Source: CAD feature listing. Evaluate the final solid. Frame: model axes, mm. A direction names the side the tool comes from. Round coordinates to 2 decimals unless told otherwise and drop trailing zeros. Loops run counter-clockwise (first coordinate to the right, second up) from the corner with the lowest first, then second, coordinate; pieces in that order, holes last. Notation, with made-up numbers: (77.25, -19.75) -> (135.25, -19.75) arc R29 ccw to (135.25, 19.25) -> close; hole circle Ø1 at (67, -36). An arc over 180 degrees is marked (long way). Put each result on its own line as item: value. Start each with the question number.
1. Set-up query: faces 4 (the flat face through (-95, -25, 187)), 5 (the flat face through (155, -25, -188)), 6 (the flat face through (-3, 141, -187.5)), 7 (the flat face through (219, 149, -100)), 8 (the flat face through (-125, -41, 175)). Return all of +Z, -Z, +X, -X, +Y, -Y with unobstructed straight access to the full face (end or side cutting, diameter ignored); none if empty.
2. Cut plane B-B (x = 125). Return the cut outline in (y, z), then the cut area to 3 significant figures.
3. Cut plane A-A (y = 305). Return the cut outline in (x, z).
4. Material intervals for L1, parallel to Z at x = 35.5, y = 98.5; L2, parallel to X at y = 119, z = 139; L3, parallel to Y at x = -0.5, z = 0, sorted ascending.
5. Cut plane D-D (z = 0). Return the cut outline in (x, y).
6. Draft query along Z for faces 1 (the flat face through (125, -50, 188)), 2 (the flat face through (0, 188, 15)), 3 (the flat face through (-3, 83, 200)). Return one class per face: pulls with the +Z half, pulls with the -Z half, needs draft (parallel to the pull), parting line crosses it, or undercut.
7. Cut plane C-C (y = -25). State how many separate pieces and enclosed holes the cut face has, then the cut area to 3 significant figures.
8. Contact query for flat-ended pins moving along their axis: pin 1 (23 mm diameter, centred on y = 305, z = 0, fed in from +X); pin 2 (1.5 mm diameter, centred on x = -73.5, z = 112.5, fed in from -Y); pin 3 (7.5 mm diameter, centred on y = -34, z = -188, fed in from +X); pin 4 (25 mm diameter, centred on x = 128.5, y = -19.5, fed in from +Z). Output: stop coordinate, or through.
```python
from build123d import *

# Parameters (mm, degrees)
SKETCH1_W           = 450
SKETCH1_H           = 400
BOSS_EXTRUDE1_DEPTH = 220
SKETCH2_W           = 425
SKETCH2_H           = 375
CUT_EXTRUDE1_DEPTH  = 160
SKETCH3_W           = 200
SKETCH3_H           = 140
CUT_EXTRUDE2_DEPTH  = 12.5
SKETCH4_W           = 30
SKETCH4_H           = 30
BOSS_EXTRUDE2_DEPTH = 260
SKETCH5_R           = 10
CUT_EXTRUDE3_DEPTH  = 30
SKETCH6_W           = 60
SKETCH6_H           = 25
BOSS_EXTRUDE3_DEPTH = 50
SKETCH7_R           = 15
CUT_EXTRUDE4_DEPTH  = 25
SKETCH8_R           = 15
CUT_EXTRUDE5_DEPTH  = 25


with BuildPart() as part:
    # Sketch1 → Boss-Extrude1 (new body)
    with BuildSketch(Plane(origin=(0, 0, 0), x_dir=(1, 0, 0), z_dir=(0, 1, 0))):
        Rectangle(SKETCH1_W, SKETCH1_H)
    extrude(amount=BOSS_EXTRUDE1_DEPTH)

    # Sketch2 → Cut-Extrude1 (cut)
    with BuildSketch(Plane(origin=(0, 220, 0), x_dir=(1, 0, 0), z_dir=(0, 1, 0))):
        Rectangle(SKETCH2_W, SKETCH2_H)
    extrude(amount=-CUT_EXTRUDE1_DEPTH, mode=Mode.SUBTRACT)

    # Sketch3 → Cut-Extrude2 (cut)
    with BuildSketch(Plane(origin=(225, 0, 0), x_dir=(0, 0, -1), z_dir=(1, 0, 0))):
        with Locations((0, 150)):
            Rectangle(SKETCH3_W, SKETCH3_H)
    extrude(amount=-CUT_EXTRUDE2_DEPTH, mode=Mode.SUBTRACT)

    # Sketch4 → Boss-Extrude2 (add)
    with BuildSketch(Plane(origin=(0, 60, 0), x_dir=(1, 0, 0), z_dir=(0, 1, 0))):
        Rectangle(SKETCH4_W, SKETCH4_H)
    extrude(amount=BOSS_EXTRUDE2_DEPTH)

    # Sketch5 → Cut-Extrude3 (cut)
    with BuildSketch(Plane(origin=(15, 0, 0), x_dir=(0, 0, -1), z_dir=(1, 0, 0))):
        with Locations((0, 305)):
            Circle(SKETCH5_R)
    extrude(amount=-CUT_EXTRUDE3_DEPTH, mode=Mode.SUBTRACT)

    # Sketch6 → Boss-Extrude3 (add)
    with BuildSketch(Plane.XZ):
        with Locations((125, 187.5)):
            Rectangle(SKETCH6_W, SKETCH6_H)
        with Locations((-125, 187.5)):
            Rectangle(SKETCH6_W, SKETCH6_H)
        with Locations((-125, -187.5)):
            Rectangle(SKETCH6_W, SKETCH6_H)
        with Locations((125, -187.5)):
            Rectangle(SKETCH6_W, SKETCH6_H)
    extrude(amount=BOSS_EXTRUDE3_DEPTH)

    # Sketch7 → Cut-Extrude4 (cut)
    with BuildSketch(Plane(origin=(0, 0, -200), x_dir=(-1, 0, 0), z_dir=(0, 0, -1))):
        with Locations((125, -25)):
            Circle(SKETCH7_R)
        with Locations((-125, -25)):
            Circle(SKETCH7_R)
    extrude(amount=-CUT_EXTRUDE4_DEPTH, mode=Mode.SUBTRACT)

    # Sketch8 → Cut-Extrude5 (cut)
    with BuildSketch(Plane.XY.offset(200)):
        with Locations((-125, -25)):
            Circle(SKETCH8_R)
        with Locations((125, -25)):
            Circle(SKETCH8_R)
    extrude(amount=-CUT_EXTRUDE5_DEPTH, mode=Mode.SUBTRACT)


solid = part.part
```
Solution:
1. face 4: +Z, -Z, -Y
1. face 5: +Z, -Z, +X, -Y
1. face 6: +Y
1. face 7: +X, +Y
1. face 8: +X, -X, -Y
2. outline: (-50, -200) -> (-40, -200) -> (-40, -175) -> (-50, -175) -> close; (-50, 175) -> (-40, 175) -> (-40, 200) -> (-50, 200) -> close; (-10, -200) -> (220, -200) -> (220, -187.5) -> (60, -187.5) -> (60, 187.5) -> (220, 187.5) -> (220, 200) -> (-10, 200) -> (-10, 175) -> (0, 175) -> (0, -175) -> (-10, -175) -> close
2. area: 29,000 mm^2
3. outline: (-15, -15) -> (15, -15) -> (15, -10) -> (-15, -10) -> close; (-15, 10) -> (15, 10) -> (15, 15) -> (-15, 15) -> close
4. L1: z = -200 to -187.5, 187.5 to 200
4. L2: x = -225 to -212.5, 212.5 to 225
4. L3: y = 0 to 295, 315 to 320
5. outline: (-225, 0) -> (225, 0) -> (225, 80) -> (212.5, 80) -> (212.5, 60) -> (15, 60) -> (15, 295) -> (-15, 295) -> (-15, 60) -> (-212.5, 60) -> (-212.5, 220) -> (-225, 220) -> close; (-15, 315) -> (15, 315) -> (15, 320) -> (-15, 320) -> close
6. face 1: needs draft
6. face 2: undercut
6. face 3: pulls with the +Z half
7. separate pieces: 8
7. enclosed holes: 0
7. area: 3,000 mm^2
8. pin 1: stops at x = 15
8. pin 2: stops at y = 0
8. pin 3: stops at x = 155
8. pin 4: stops at z = 200
